Input: part model. Units: mm. Frame: model coordinates. Give positions to 0.01 mm unless a question says otherwise; leave off trailing zeros. Loops run counter-clockwise (first coordinate to the right, second up) from the corner with the lowest first, then second, coordinate; pieces in that order, holes last. Notation, with made-up numbers: M -2,54 L 9,54 A35 cw 9,86 Z; hole C 49,78 d3. An arc over 180 degrees is marked long. Answer as a JSON object with one key per item and string values. Group by question number.
1) Draft query along Z for faces 1 (the flat face through (0.085, 0, 0)), 2 (the cylindrical face through (4.59, 1.05, 0.33)). Return one class per face: +Z half, -Z half, draft (parallel to the pull), parting line (faces both ways), or undercut.
2) Ray query, L1, parallel to Z at x = 8.75, y = 0.2; L2, parallel to Y at x = 2, z = 0.3; L3, parallel to Z at x = 3.5, y = 0.1. Return the intervals inside material, ascending.
3) First-contact query: P1, Ø2, axis at x = 7, z = -1, coming from the -Y side; P2, Ø1.5, axis at x = 7.5, y = -1.5, coming from the +Z side; P3, Ø1, axis at x = 3.5, y = 0, coming from the +Z side. Flat tips, straight axial feed; report the tip coordinate or a pass-through.
4) Section query A-A on x = 7.75. Return loops of the section in (y, z) (1 decimal).
Solid Edge part; units mm, degrees
sketch "Sketch1" plane through (0, 0, 0) normal (0, 0, 1) x (1, 0, 0)
  line L0 (-0.7, 0) -> (-0.7, 2.15)
  line L1 (-0.7, 2.15) -> (0.0487, 2.15)
  line L2 (0.0487, 2.15) -> (1.3, 1.1)
  line L3 (1.3, 1.1) -> (7.5, 1.1)
  line L4 (7.5, 1.1) -> (9.5, 0)
  line L5 (9.5, 0) -> (-0.7, 0)
revolve "RevolvedProtrusion1" add sketch "Sketch1" angle 360 about axis through (9.5, 0, 0) along (-1, 0, 0)
cosmetic_thread "Thread1"
sketch "Sketch2" plane through (0, 0, 0) normal (0, 0, 1) x (1, 0, 0)
  line L0 (-0.83, 0) -> (-0.83, 2.365)
  line L1 (-0.83, 2.365) -> (0, 2.365)
  line L2 (0, 2.365) -> (0, 2.15)
  arc A0 (0, 2.15) -> (-0.7, 0) centre (2.9518, 0) ccw
  line L3 (-0.7, 0) -> (-0.83, 0)
revolve "RevolvedCutout1" cut sketch "Sketch2" angle 360 about axis through (-0.7, 0, 0) along (-1, 0, 0)
sketch "Sketch3" plane through (0, 0, 0) normal (0, 0, 1) x (1, 0, 0)
  line L0 (0.9, 0.9) -> (1.7, 0.9)
  line L1 (1.7, 0.9) -> (1.7, 1.1)
  line L2 (1.7, 1.1) -> (1.5912, 1.1)
  arc A0 (1.5912, 1.1) -> (1.0769, 1.2872) centre (1.5912, 1.9) cw
  line L3 (1.0769, 1.2872) -> (0.9, 1.4356)
  line L4 (0.9, 1.4356) -> (0.9, 0.9)
revolve "RevolvedProtrusion2" add sketch "Sketch3" angle 360 about axis through (1.7, 0, 0) along (-1, 0, 0)
sketch "Sketch4" plane through (-0.7, 0, 0) normal (1, 0, 0) x (0, 1, 0)
  line L0 (-0.35, 1.4) -> (-0.2765, 0.56)
  line L1 (-0.2765, 0.56) -> (-0.35, 0.35)
  line L2 (-0.35, 0.35) -> (-0.56, 0.2765)
  line L3 (-0.56, 0.2765) -> (-1.4, 0.35)
  line L4 (-1.4, 0.35) -> (-1.4, -0.35)
  line L5 (-1.4, -0.35) -> (-0.56, -0.2765)
  line L6 (-0.56, -0.2765) -> (-0.35, -0.35)
  line L7 (-0.35, -0.35) -> (-0.2765, -0.56)
  line L8 (-0.2765, -0.56) -> (-0.35, -1.4)
  line L9 (-0.35, -1.4) -> (0.35, -1.4)
  line L10 (0.35, -1.4) -> (0.2765, -0.56)
  line L11 (0.2765, -0.56) -> (0.35, -0.35)
  line L12 (0.35, -0.35) -> (0.56, -0.2765)
  line L13 (0.56, -0.2765) -> (1.4, -0.35)
  line L14 (1.4, -0.35) -> (1.4, 0.35)
  line L15 (1.4, 0.35) -> (0.56, 0.2765)
  line L16 (0.56, 0.2765) -> (0.35, 0.35)
  line L17 (0.35, 0.35) -> (0.2765, 0.56)
  line L18 (0.2765, 0.56) -> (0.35, 1.4)
  line L19 (0.35, 1.4) -> (-0.35, 1.4)
extrude "ExtrudedCutout_1" cut sketch "Sketch4" against normal blind 0.785 and the other way blind 0.785
properties part number "Tapping screw DIN 7983 ST2.2x9.5-C-H 55690.022.009(High)"
Output:
{
 "1": {"face 1": "undercut", "face 2": "parting line"},
 "2": {"L1": "z = -0.36 to 0.36", "L2": "y = -1.06 to 1.06", "L3": "z = -1.1 to 1.1"},
 "3": {"P1": "stops at y = -1.1", "P2": "stops at z = 0.8", "P3": "stops at z = 1.1"},
 "4": {"outline": "C 0,0 d1.9"}
}
